CAD build for the part. Positions are in the model's coordinates, mm. A direction names the side the tool comes from. Coordinates: 2 decimals unless noted, no trailing zeros. Loops run counter-clockwise (first coordinate to the right, second up) from the corner with the lowest first, then second, coordinate; pieces in that order, holes last.
1) Wall check: line 1 along Y through (x, z) = (-26.5, 2.8); line 2 along Z through (x, y) = (15.5, 10.7); line 3 along Z through (x, y) = (7.5, 3). Give the ranges that are in metal, low to high.
2) Saw through at D-D, the plane y = 13.25. Write the cut outline in (x, z).
3) Saw through at C-C, the plane x = 0. Write the cut outline in (y, z), and give its area (3 significant figures).
4) Saw through at A-A, the plane z = 40. Write the cut outline in (x, y), and give its area (3 significant figures).
5) Which spindle directions (+Z, -Z, +X, -X, +Y, -Y) get a long thin tool onto all of the face, cutting with end or side? Do faces 4 (the cylindrical face through (-24.354, -2.324, 2.028)), 5 (the flat face through (-29, -6, 7)), 6 (the flat face through (-21, 11, 23)), 7 (the flat face through (21, 11, 23)), 8 (the cylindrical face through (30.077, -1.874, 5.521)). Say none if no direction does.
6) Two-plate mould, pull along Y, no slides. Class faces 1 (the cylindrical face through (15.272, 11.958, 10.735)), 2 (the flat face through (0, 15, 12)), 3 (the flat face through (-25, -5, 4)): +Y half, -Y half, draft (parallel to the pull), parting line (faces both ways), or undercut.
7) Saw through at B-B, the plane y = -3. Write the cut outline in (x, z), and give its area (3 significant figures).
8) Pin check, flat tips, straight feed: pin 1 Ø5 at (x, y) = (26.5, 2) entering from +Z; pin 2 Ø6 at (x, y) = (-26.5, -3) entering from +Z; pin 3 Ø5.5 at (x, z) = (15.5, 40) entering from -Y; pin 4 Ø3 at (x, z) = (-15.5, 9) entering from -Y (3 decimals). Stop position of each tip, or through.
```python
from build123d import *

# Parameters (mm, degrees)
SKETCH_W        = 42
SKETCH_H        = 30
PAD_DEPTH       = 4
SKETCH001_W     = 42
SKETCH001_H     = 6
PAD001_DEPTH    = 42
SKETCH002_R     = 12.5
POCKET_DEPTH    = 6
SKETCH003_R     = 1.75
POCKET001_DEPTH = 6
SKETCH004_W     = 23
SKETCH004_H     = 7
PAD002_DEPTH    = 11
SKETCH005_W     = 23
SKETCH005_H     = 7
PAD003_DEPTH    = 11
SKETCH006_R     = 2.25
POCKET002_DEPTH = 10
SKETCH007_R     = 3.75
POCKET003_DEPTH = 3
FILLET_R        = 1


with BuildPart() as part:
    # Sketch → Pad (new body)
    with BuildSketch(Plane.XY):
        Rectangle(SKETCH_W, SKETCH_H)
    extrude(amount=PAD_DEPTH)

    # Sketch001 (on Face6 of Pad) → Pad001 (join)
    with BuildSketch(Plane.XY.offset(4)):
        with Locations((0, 12)):
            Rectangle(SKETCH001_W, SKETCH001_H)
    extrude(amount=PAD001_DEPTH)

    # Sketch002 (on Face7 of Pad001) → Pocket (cut)
    with BuildSketch(Plane(origin=(0, 15, 0), x_dir=(-1, 0, 0), z_dir=(0, 1, 0))):
        with Locations((0, 25)):
            Circle(SKETCH002_R)
    extrude(amount=-POCKET_DEPTH, mode=Mode.SUBTRACT)

    # Sketch003 (on Face6 of Pocket) → Pocket001 (cut)
    with BuildSketch(Plane.XZ.offset(-9)):
        with Locations((15.5, 9)):
            Circle(SKETCH003_R)
        with Locations((-15.5, 9)):
            Circle(SKETCH003_R)
        with Locations((15.5, 40)):
            Circle(SKETCH003_R)
        with Locations((-15.5, 40)):
            Circle(SKETCH003_R)
    extrude(amount=-POCKET001_DEPTH, mode=Mode.SUBTRACT)

    # Sketch004 (on Face2 of Pocket001) → Pad002 (join)
    with BuildSketch(Plane(origin=(-21, 0, 0), x_dir=(0, -1, 0), z_dir=(-1, 0, 0))):
        with Locations((3.5, 3.5)):
            Rectangle(SKETCH004_W, SKETCH004_H)
    extrude(amount=PAD002_DEPTH)

    # Sketch005 (on Face1 of Pad002) → Pad003 (join)
    with BuildSketch(Plane.YZ.offset(21)):
        with Locations((-3.5, 3.5)):
            Rectangle(SKETCH005_W, SKETCH005_H)
    extrude(amount=PAD003_DEPTH)

    # Sketch006 (on Face19 of Pad003) → Pocket002 (cut)
    with BuildSketch(Plane.XY.offset(7)):
        with Locations((-26.5, -3)):
            Circle(SKETCH006_R)
        with Locations((26.5, -3)):
            Circle(SKETCH006_R)
    extrude(amount=-POCKET002_DEPTH, mode=Mode.SUBTRACT)

    # Sketch007 (on Face23 of Pocket002) → Pocket003 (cut)
    with BuildSketch(Plane.XY.offset(7)):
        with Locations((-26.5, -3)):
            Circle(SKETCH007_R)
        with Locations((26.5, -3)):
            Circle(SKETCH007_R)
    extrude(amount=-POCKET003_DEPTH, mode=Mode.SUBTRACT)

    # Fillet
    fillet_edges = [part.edges().sort_by_distance(p)[0] for p in [
        (-21, -3.5, 7),
        (21, -3.5, 7),
        (21, -3.5, 4),
        (-21, -3.5, 4),
    ]]
    fillet(fillet_edges, radius=FILLET_R)


solid = part.part
```
Data:
1. line 1: y = -15 to -5.25, -0.75 to 8
1. line 2: z = 0 to 7.25, 10.75 to 38.25, 41.75 to 46
1. line 3: z = 0 to 4
2. outline: (-21, 0) - (21, 0) - (21, 46) - (-21, 46) - close; hole circle Ø3.5 at (-15.5, 9); hole circle Ø3.5 at (-15.5, 40); hole circle Ø25 at (0, 25); hole circle Ø3.5 at (15.5, 9); hole circle Ø3.5 at (15.5, 40)
3. outline: (-15, 0) - (15, 0) - (15, 12.5) - (9, 12.5) - (9, 4) - (-15, 4) - close; (9, 37.5) - (15, 37.5) - (15, 46) - (9, 46) - close
3. area: 222 mm2
4. outline: (-21, 9) - (-17.25, 9) - (-17.25, 15) - (-21, 15) - close; (-13.75, 9) - (13.75, 9) - (13.75, 15) - (-13.75, 15) - close; (17.25, 9) - (21, 9) - (21, 15) - (17.25, 15) - close
4. area: 210 mm2
5. face 4: +Z, -Z
5. face 5: +Z, +X, -X, +Y, -Y
5. face 6: +Z, -Z, -X, +Y
5. face 7: +Z, -Z, +X, +Y
5. face 8: +Z
6. face 1: draft
6. face 2: +Y half
6. face 3: undercut
7. outline: (-32, 0) - (-28.75, 0) - (-28.75, 4) - (-30.25, 4) - (-30.25, 7) - (-32, 7) - close; (-24.25, 0) - (24.25, 0) - (24.25, 4) - (22.75, 4) - (22.75, 7) - (22, 7) arc R1 ccw to (21, 6) - (21, 5) arc R1 cw to (20, 4) - (-20, 4) arc R1 cw to (-21, 5) - (-21, 6) arc R1 ccw to (-22, 7) - (-22.75, 7) - (-22.75, 4) - (-24.25, 4) - close; (28.75, 0) - (32, 0) - (32, 7) - (30.25, 7) - (30.25, 4) - (28.75, 4) - close
7. area: 241 mm2
8. pin 1: stops at z = 7
8. pin 2: stops at z = 4
8. pin 3: stops at y = 9
8. pin 4: passes through
